Input: part model. Units: mm. Frame: model coordinates. A direction names the side the tool comes from. Coordinates: 2 decimals unless noted, no trailing zeros. Order: outer loops, then holes, each group sorted by start corner. A loop starts at its lowest first (then second) coordinate and runs counter-clockwise, first axis right, second up. Notation, with made-up numbers: (-11.5, 53) -> (23.5, 53) arc R13 cw to (23.5, 78) -> close; hole circle Ø5 at (-2, 16). An arc over 180 degrees is marked (long way). Use one line per item in the form item = value. Start each with the question number.
1) Section query B-B on x = 16. Output: boundary loops of the cut face in (y, z), then the cut area to 3 significant figures.
2) Section query D-D on x = 1.5. Output: boundary loops of the cut face in (y, z).
3) Access query for faces 1 (the cylindrical face through (6.81, 3.5, 0.99)), 2 (the flat face through (30.403, 7.618, 15.194)), 3 (the flat face through (-5.32, 0.85, 1.51)). Directions: +Z, -Z, +X, -X, +Y, -Y. A direction counts if a zero-diameter tool reaches every point of the face in a straight line with its end or side. Return the directions, or none.
4) Section query A-A on x = 45.9. Output: boundary loops of the cut face in (y, z), then the cut area to 3 significant figures.
5) Draft query along Z for faces 4 (the cylindrical face through (5.715, 26.636, 0.986)), 5 (the flat face through (25, 15, 2)), 6 (the flat face through (26.07, 27.6, 47.84)). Return one class per face: pulls with the +Z half, pulls with the -Z half, needs draft (parallel to the pull), parting line crosses it, or undercut.
6) Ray query, line 1 along Y through (x, z) = (5.5, 1.45); line 2 along Z through (x, y) = (21, 21.5); line 3 along Z through (x, y) = (32.5, 11). Return the intervals inside material, ascending.
7) Section query C-C on y = 18. Count the separate pieces of the cut face and the enclosed holes in it, then the cut area to 3 significant figures.
8) Pin query (flat end, axial travel): pin 1 (14 mm diameter, centred on y = 20.5, z = 34, fed in from +X); pin 2 (12 mm diameter, centred on x = 9.5, y = 12, fed in from +Z); pin 3 (1.6 mm diameter, centred on y = 13, z = 1, fed in from -X). Return the tip coordinate at first contact, or that it passes through.
from build123d import *

# Parameters (mm, degrees)
SKETCH1_W           = 51.4
SKETCH1_H           = 30
BOSS_EXTRUDE1_DEPTH = 2
SKETCH2_R           = 1.65
CUT_EXTRUDE1_DEPTH  = 10
SKETCH3_W           = 49.5
SKETCH3_H           = 53.5
BOSS_EXTRUDE2_DEPTH = 2
FILLET1_R           = 24
SKETCH5_R           = 2.25
CUT_EXTRUDE2_DEPTH  = 2
SKETCH6_R           = 20
CUT_EXTRUDE3_DEPTH  = 2


with BuildPart() as part:
    # Sketch1 → Boss-Extrude1 (new body)
    with BuildSketch(Plane.XY):
        with Locations((25.7, 15)):
            Rectangle(SKETCH1_W, SKETCH1_H)
    extrude(amount=BOSS_EXTRUDE1_DEPTH)

    # Sketch2 → Cut-Extrude1 (cut)
    with BuildSketch(Plane(origin=(0, 0, 0), x_dir=(-1, 0, 0), z_dir=(0, 0, -1))):
        with Locations((-45.9, 25)):
            Circle(SKETCH2_R)
        with Locations((-5.5, 25)):
            Circle(SKETCH2_R)
        with Locations((-5.5, 4.5)):
            Circle(SKETCH2_R)
        with Locations((-45.9, 4.5)):
            Circle(SKETCH2_R)
    extrude(amount=-CUT_EXTRUDE1_DEPTH, mode=Mode.SUBTRACT)

    # Sketch3 → Boss-Extrude2 (add)
    with BuildSketch(Plane(origin=(0, -0.8660254037844364, 0.4999999999999961), x_dir=(1, 0, 0), z_dir=(0, -0.8660254037844398, 0.499999999999998))):
        with Locations((14.25, 28.482050808)):
            Rectangle(SKETCH3_W, SKETCH3_H)
    extrude(amount=-BOSS_EXTRUDE2_DEPTH)

    # Fillet1
    fillet1_edges = [part.edges().sort_by_distance(p)[0] for p in [
        (-10.5, 27.616025404, 47.832359102),
    ]]
    fillet(fillet1_edges, radius=FILLET1_R)

    # Sketch5 → Cut-Extrude2 (cut)
    with BuildSketch(Plane(origin=(0, -0.8660254037844378, 0.4999999999999969), x_dir=(1, 0, 0), z_dir=(0, -0.8660254037844399, 0.49999999999999806))):
        with Locations(Location((35.9, 49.210750739, 0), (0, 0, 270))):
            Circle(SKETCH5_R)
        with Locations(Location((-7.1, 11.210750739, 0), (0, 0, 270))):
            Circle(SKETCH5_R)
    extrude(amount=-CUT_EXTRUDE2_DEPTH, mode=Mode.SUBTRACT)

    # Sketch6 → Cut-Extrude3 (cut)
    with BuildSketch(Plane(origin=(0, -0.8660254037844378, 0.4999999999999969), x_dir=(1, 0, 0), z_dir=(0, -0.8660254037844399, 0.49999999999999806))):
        with Locations(Location((12.9, 29.210750739, 0), (0, 0, 270))):
            Circle(SKETCH6_R)
    extrude(amount=-CUT_EXTRUDE3_DEPTH, mode=Mode.SUBTRACT)


solid = part.part
Answers below:
q1.outline = (0, 0) -> (30, 0) -> (30, 2) -> (2.31, 2) -> (5.59, 7.69) -> (3.86, 8.69) -> (0, 2) -> close; (23.62, 42.91) -> (25.35, 41.91) -> (28.48, 47.33) -> (26.75, 48.33) -> close
q1.area = 86.8 mm^2
q2.outline = (0, 0) -> (30, 0) -> (30, 2) -> (2.31, 2) -> (7.25, 10.57) -> (5.52, 11.57) -> (0, 2) -> close; (21.96, 40.03) -> (23.69, 39.03) -> (26.87, 44.55) -> (25.14, 45.55) -> close
q3.face_1 = -Z
q3.face_2 = +Z, +X, -X, -Y
q3.face_3 = -Z, -X, -Y
q4.outline = (0, 0) -> (2.85, 0) -> (2.85, 2) -> (0, 2) -> close; (6.15, 0) -> (23.35, 0) -> (23.35, 2) -> (6.15, 2) -> close; (26.65, 0) -> (30, 0) -> (30, 2) -> (26.65, 2) -> close
q4.area = 46.8 mm^2
q5.face_4 = needs draft
q5.face_5 = undercut
q5.face_6 = pulls with the +Z half
q6.line_1 = 0 to 2.85, 6.15 to 23.35, 26.65 to 30
q6.line_2 = 0 to 2
q6.line_3 = 0 to 2, 17.05 to 21.05
q7.separate_pieces = 3
q7.enclosed_holes = 0
q7.area = 149 mm^2
q8.pin_1 = 39
q8.pin_2 = 2
q8.pin_3 = 0
